The listing builds one solid part. Answer for the finished solid, in the listing's coordinates (mm). A direction names the side the tool comes from. Round coordinates to 2 decimals unless told otherwise and drop trailing zeros. Write each loop counter-clockwise with the first axis right and the second up, starting at its lowest first coordinate (ties: lowest second). Pieces come first, ordered by that corner, then holes. Notation, with made-up numbers: (58.25, 82) - (65.25, 82) arc R24 cw to (65.25, 99) - close; hole circle Ø8 at (-35.5, 18). An arc over 180 degrees is marked (long way). Answer as CSV lines item,"result". Start each with the question number.
Item 1: A cutting plane is placed at D-D on z = 73.5. Determine the outline of the cut face in (x, y).
Item 2: For a pull along X with two mould halves and no side action, classify faces 1 (the flat face through (8.71, 18, 58)), 2 (the flat face through (48, 9.779, 89)), 3 (the flat face through (31, 11, 100)) as pulls with the +X half, pulls with the -X half, needs draft (parallel to the pull), parting line crosses it, or undercut.
Item 3: A cutting plane is placed at C-C on x = 40.5. Determine the outline of the cut face in (y, z).
Item 4: Straight lines are drawn through the part: line 1 along X through (y, z) = (13.5, 71); line 2 along Y through (x, z) = (27.5, 23); line 3 along X through (y, z) = (19, 13.5). For each, find the intervals that lie inside material, in ascending order. Write a range as [from, to].
Item 5: Flat-ended cylindrical pins translate along their axes: pin 1 (3 mm diameter, centred on x = 37.5, z = 21, fed in from +Y); pin 2 (8 mm diameter, centred on x = 47.88, z = 88.8, fed in from +Y); pin 3 (2.5 mm diameter, centred on x = 49, z = 89, fed in from -Y); pin 4 (1.5 mm diameter, centred on x = 11.5, y = 20, fed in from -Z). Find the tip coordinate at first contact, or state that the pin passes through.
Item 6: A cutting plane is placed at B-B on z = 17. Determine the outline of the cut face in (x, y).
Item 7: A cutting plane is placed at A-A on y = 24.75. Determine the outline of the cut face in (x, z), and give its area (3 significant figures).
Item 8: Which of the six approach directions +Z, -Z, +X, -X, +Y, -Y give full straight-line access (tool end or side, diameter ignored) to faces 4 (the flat face through (11, 20, 35)), 5 (the flat face through (51, 27.779, 47)), 6 (the cylindrical face through (49.22, 8.77, 90.91)), 7 (the flat face through (48.71, 20, 47))?
Autodesk Inventor part; units mm, degrees
ref_plane "YZ Plane" through (0, 0, 0) normal (1, 0, 0) x (0, 1, 0)
ref_plane "XZ Plane" through (0, 0, 0) normal (0, 1, 0) x (-1, 0, 0)
ref_plane "XY Plane" through (0, 0, 0) normal (0, 0, 1) x (1, 0, 0)
sketch "Sketch1" plane through (0, 0, 0) normal (0, 0, 1) x (1, 0, 0)
  line L0 (13.7104, 12.7791) -> (48.7104, 12.7791)
  line L1 (48.7104, 12.7791) -> (48.7104, 27.7791)
  line L2 (13.7104, 12.7791) -> (13.7104, 27.7791)
  line L3 (8.7104, 27.7791) -> (8.7104, 7.7791)
  line L4 (8.7104, 7.7791) -> (53.7104, 7.7791)
  line L5 (53.7104, 7.7791) -> (53.7104, 27.7791)
  line L6 (8.7104, 27.7791) -> (13.7104, 27.7791)
  line L7 (48.7104, 27.7791) -> (53.7104, 27.7791)
  point P0 (0, 0)
  dimension "d0" = 35
  dimension "d1" = 15
  dimension "d2" = 15
  dimension "d3" = 5
extrude "Extrusion1" add sketch "Sketch1" along normal blind 100 and the other way blind 5
sketch "Sketch2" plane through (8.7104, 7.7791, -5) normal (0, -1, 0) x (1, 0, 0)
  circle A0 centre (39.17, 93.8) radius 2.5
  line L0 (45, 0) -> (45, 105)
  line L1 (0, 105) -> (45, 105)
  point P0 (-8.7104, 5)
  dimension "d6" = 5
  dimension "d7" = 5.83
  dimension "d8" = 11.2
extrude "Extrusion2" cut sketch "Sketch2" against normal blind 2
sketch "Sketch3" plane through (8.7104, 7.7791, 100) normal (-1, 0, 0) x (0, 0, 1)
  line L0 (-105, 20) -> (-105, 5)
  line L1 (-105, 5) -> (0, 5)
  line L2 (-105, 20) -> (-105, 5)
  line L3 (-105, 5) -> (-65, 5)
  line L4 (-65, 5) -> (-65, 20)
  line L5 (-65, 20) -> (-105, 20)
  point P0 (-100, -7.7791)
  dimension "d13" = 40
extrude "Extrusion3" cut sketch "Sketch3" against normal blind 10
sketch "Sketch4" plane through (0, 0, -5) normal (0, 0, -1) x (-1, 0, 0)
  line L0 (-53.7104, 27.7791) -> (-53.7104, 7.7791)
  line L1 (-53.7104, 7.7791) -> (-8.7104, 7.7791)
  line L2 (-17.7104, 42.7791) -> (-17.7104, 46.7534)
  line L3 (-17.7104, 46.7534) -> (-53.7104, 46.7534)
  line L4 (-53.7104, 46.7534) -> (-53.7104, 7.7791)
  line L5 (-48.7104, 12.7791) -> (-13.7104, 12.7791)
  line L6 (-10.7104, 42.7791) -> (-10.7104, 41.7534)
  line L7 (-10.7104, 41.7534) -> (-48.7104, 41.7534)
  line L8 (-48.7104, 41.7534) -> (-48.7104, 12.7791)
  line L9 (-17.7104, 42.7791) -> (-10.7104, 42.7791)
  line L10 (-8.7104, 12.7791) -> (-13.7104, 12.7791)
  line L11 (-13.7104, 12.7791) -> (-8.7104, 12.7791)
  line L12 (-8.7104, 12.7791) -> (-8.7104, 7.7791)
  line L13 (-17.7104, 42.7791) -> (-17.7104, 41.7534)
  point P0 (0, 0)
  point P1 (-17.7104, 44.7534)
  dimension "d16" = 36
  dimension "d17" = 40
  dimension "d18" = 5
  dimension "d19" = 30
ref_plane "Work Plane1" through (0, 0, -1) normal (0, 0, -1) x (-1, 0, 0)
sketch "Sketch5" plane through (0, 0, -1) normal (0, 0, -1) x (-1, 0, 0)
  line L0 (-8.7104, 12.7791) -> (-13.7104, 12.7791)
  line L1 (-48.7104, 27.7791) -> (-48.7104, 12.7791)
  line L2 (-8.7104, 12.7791) -> (-8.7104, 7.7791)
  line L3 (-8.7104, 12.7791) -> (-8.7104, 7.7791)
  line L4 (-8.7104, 7.7791) -> (-53.7104, 7.7791)
  line L5 (-8.7104, 7.7791) -> (-53.7104, 7.7791)
  line L6 (-53.7104, 7.7791) -> (-53.7104, 12.7791)
  line L7 (-53.7104, 12.7791) -> (-8.7104, 12.7791)
  point P0 (0, 0)
  point P1 (-48.7104, 41.7534)
  point P2 (-10.7104, 9.7791)
extrude "Extrusion6" add sketch "Sketch5" along normal blind 4
equation "\"BendRadius\" = Thickness"
equation "\"BendReliefWidth\" = Thickness"
equation "\"BendReliefDepth\" = 0.5 * Thickness"
equation "\"CornerReliefSize\" = 4 * Thickness"
equation "\"MinimumRemnant\" = 2 * Thickness"
equation "\"TransitionRadius\" = BendRadius"
equation "\"JacobiRadiusSize\" = BendRadius"
properties part number "inslide"
Geometry says:
1,outline,"(8.71, 7.78) - (53.71, 7.78) - (53.71, 27.78) - (48.71, 27.78) - (48.71, 12.78) - (13.71, 12.78) - (13.71, 27.78) - (8.71, 27.78) - close"
2,face 1,"pulls with the -X half"
2,face 2,"undercut"
2,face 3,"needs draft"
3,outline,"(7.78, -5) - (12.78, -5) - (12.78, 100) - (7.78, 100) - close"
4,line 1,"x = [8.71, 13.71], [48.71, 53.71]"
4,line 2,"y = [7.78, 12.78]"
4,line 3,"x = [48.71, 53.71]"
5,pin 1,"stops at y = 12.78"
5,pin 2,"stops at y = 27.78"
5,pin 3,"stops at y = 9.78"
5,pin 4,"stops at z = 35"
6,outline,"(8.71, 7.78) - (53.71, 7.78) - (53.71, 27.78) - (48.71, 27.78) - (48.71, 12.78) - (8.71, 12.78) - close"
7,outline,"(8.71, 35) - (13.71, 35) - (13.71, 100) - (8.71, 100) - close; (48.71, -5) - (53.71, -5) - (53.71, 100) - (48.71, 100) - close"
7,area,"850 mm^2"
8,face 4,"-Z, -X, +Y"
8,face 5,"+Z, -Z, +X, -X, +Y"
8,face 6,"-Y"
8,face 7,"+Z, -Z, +Y"
